Can you work these out from the model? Positions are in its coordinate system, mm. Coordinates: 2 decimals unless noted, no trailing zeros. Loops run counter-clockwise (first coordinate to the right, second up) from the corner with the lowest first, then second, coordinate; pieces in that order, holes last. Notation, with made-up numbers: M 36.25,32.5 L 49.25,32.5 A12 ccw 49.25,43.5 Z; hole C 83.25,-13.5 d5. An arc over 180 degrees is marked long. Answer as a JSON object with one key per item and string values. Group by question number.
Item 1: If I drill on line 1 (Z direction, x = 127, y = -1.5); line 2 (Z direction, x = 88.5, y = -2.5); line 3 (Z direction, x = 155, y = -7), over which ranges is the centre line in solid material (lowest first)?
Item 2: Suppose I cut it at B-B (z = -61). Write out the boundary of the cut face in (x, y), then the cut area to 3 significant figures.
Item 3: Suppose I cut it at A-A (y = -12). Write out the boundary of the cut face in (x, z), then the cut area to 3 significant figures.
Item 4: I'm going to push flat-ended pins straight in: pin 1 Ø6 at (x, z) = (153.5, -8.5) entering from +Y; pin 2 Ø1.5 at (x, z) = (91.5, -52.5) entering from +Y; pin 3 Ø3 at (x, y) = (89, -6) entering from -Z. Where does each tip first touch, or does it pass through?
Item 5: We'd pull the mould along Z, two halves only. Please class faces 1 (the flat face through (41, 0, -54)), 2 (the flat face through (103.02, -9.32, -54.2)), 3 (the conical face through (202.98, -3.49, -28.79)): +Z half, -Z half, draft (parallel to the pull), parting line (faces both ways), or undercut.
```python
from build123d import *

# Parameters (mm, degrees)
BOSS_EXTRUDE1_DEPTH     = 19.05
BOSS_EXTRUDE1_DRAFT     = 29.55
CUT_EXTRUDE1_DEPTH      = 226.867324057
CUT_EXTRUDE1_DEPTH_BACK = 226.867324057
SKETCH2_OUTSIDE_W       = 274.774
SKETCH2_OUTSIDE_H       = 69.024
SKETCH2_OUTSIDE_W_2     = 203.2
SKETCH2_OUTSIDE_H_2     = 18.896108653
SKETCH4_R               = 19.414391595
CUT_EXTRUDE2_DEPTH      = 212.8485235
CUT_EXTRUDE2_TAPER      = -10.5


with BuildPart() as part:
    # Sketch1 → Boss-Extrude1 (with draft: the straight prism first)
    with BuildSketch(Plane(origin=(0, 0, 0), x_dir=(1, 0, 0), z_dir=(0, 1, 0))):
        Polygon((0, 0), (203.2, 17.777696428), (203.2, 40.129696428), (0, 57.907392857), align=None)
    extrude(amount=-BOSS_EXTRUDE1_DEPTH)
    # Boss-Extrude1: the draft: its side faces are tilted about the plane it starts from
    boss_extrude1_sides = [part.faces().sort_by_distance(p)[0] for p in [
        (101.6, -9.525, -8.888848214),
        (203.2, -9.525, -28.953696428),
        (101.6, -9.525, -49.018544643),
        (0, -9.525, -28.953696428),
    ]]
    draft(boss_extrude1_sides, Plane(origin=(0, 0, 0), x_dir=(1, 0, 0), z_dir=(0, 1, 0)), BOSS_EXTRUDE1_DRAFT)

    # Sketch2 outside → Cut-Extrude1 (cut, two sides: drawn at the far end of the back side and taken through both)
    with BuildSketch(Plane.XY.offset(-CUT_EXTRUDE1_DEPTH_BACK)):
        with Locations((101.6, -9.525)):
            Rectangle(SKETCH2_OUTSIDE_W, SKETCH2_OUTSIDE_H)
        with Locations((101.6, -9.448054327)):
            Rectangle(SKETCH2_OUTSIDE_W_2, SKETCH2_OUTSIDE_H_2, mode=Mode.SUBTRACT)
    extrude(amount=CUT_EXTRUDE1_DEPTH + CUT_EXTRUDE1_DEPTH_BACK, mode=Mode.SUBTRACT)

    # Sketch4 → Cut-Extrude2 (cut)
    with BuildSketch(Plane(origin=(197.664687281, -33.077724493, 0), x_dir=(0, 0, -1), z_dir=(0.9862856015372313, -0.16504760586067801, 0))):
        with Locations((28.953696428, 49.412673511)):
            Circle(SKETCH4_R)
    extrude(amount=-CUT_EXTRUDE2_DEPTH, taper=CUT_EXTRUDE2_TAPER, mode=Mode.SUBTRACT)

    # Cut-Extrude2 cone 1 section (through the dimple's axis) → Cut-Extrude2 other way (revolve, cut)
    with BuildSketch(Plane(origin=(205.820130743, 15.657283924, -28.953696428), x_dir=(0, 0, 1), z_dir=(0.165047606, 0.986285602, 0))):
        Polygon((0, 0), (19.414391595, 0), (0, 116.01582945), align=None)
    revolve(axis=Axis((205.820130743, 15.657283924, -28.953696428), (0.986285602, -0.165047606, 0)), mode=Mode.SUBTRACT)


solid = part.part
```
From the geometry:
{
 "1": {"line 1": "-47.65 to -43.54, -14.36 to -10.26", "line 2": "-51.59 to -44.29, -13.61 to -6.32", "line 3": "-48.33 to -9.58"},
 "2": {"outline": "M 0,-18.9 L 87.57,-18.9 L 0,-5.43 Z", "area": "589 mm2"},
 "3": {"outline": "M 0,-64.74 L 203.2,-46.96 L 203.2,-10.95 L 0,6.83 Z", "area": "10,900 mm2"},
 "4": {"pin 1": "y = -3.37", "pin 2": "y = -3.24", "pin 3": "z = -54.4"},
 "5": {"face 1": "draft", "face 2": "-Z half", "face 3": "undercut"}
}
